Could you check a few things on this drawing? It's one solid part, dimensions in mm from its lowest x, y, z. A direction names the side the tool comes from. Round coordinates to 2 decimals unless told otherwise and drop trailing zeros. Write each loop counter-clockwise with the first axis right and the second up, starting at its lowest first coordinate (ties: lowest second). Pieces come first, ordered by that corner, then holes. Notation, with made-up numbers: M 44,-11 L 97,-11 A5 ccw 97,-4 Z; hole C 62.5,74 d4. An arc over 180 degrees is marked long. One line per item, written item: value. Start each with the question number.
(1) I want a section at B-B on z = 46. Please give me the cut outline in (x, y), and give its area (3 significant figures).
(2) I'm going to push flat-ended pins straight in: pin 1 Ø12.5 at (y, z) = (17, 46) entering from +X; pin 2 Ø2 at (x, y) = (60, 46.5) entering from +Z. Where does each tip first touch, or does it pass through?
(3) Which directions (+Z, -Z, +X, -X, +Y, -Y) give clear straight access to the entire face, cutting with the end or side of a thin tool? Please do the marked faces 1, 2 and 3.
(4) I want a section at D-D on z = 131. Please give me the cut outline in (x, y) (1 decimal).
(5) Thinking about a two-plate mould opening in Z: for the marked faces 4, 5 and 6, which applies, released by +Z, released by -Z, zero draft, split by the parting line, or undercut?
(6) I want a section at A-A on y = 95. Please give me the cut outline in (x, z).
(7) If I drill on L1, parallel to X at y = 68, z = 16; L2, parallel to Z at x = 15, y = 44.5 (1 decimal); L3, parallel to Z at x = 20, y = 40.5 (1 decimal), over which ranges is the centre line in solid material (lowest first)?
(8) I want a section at C-C on x = 84. Please give me the cut outline in (y, z), and give its area (3 significant figures).
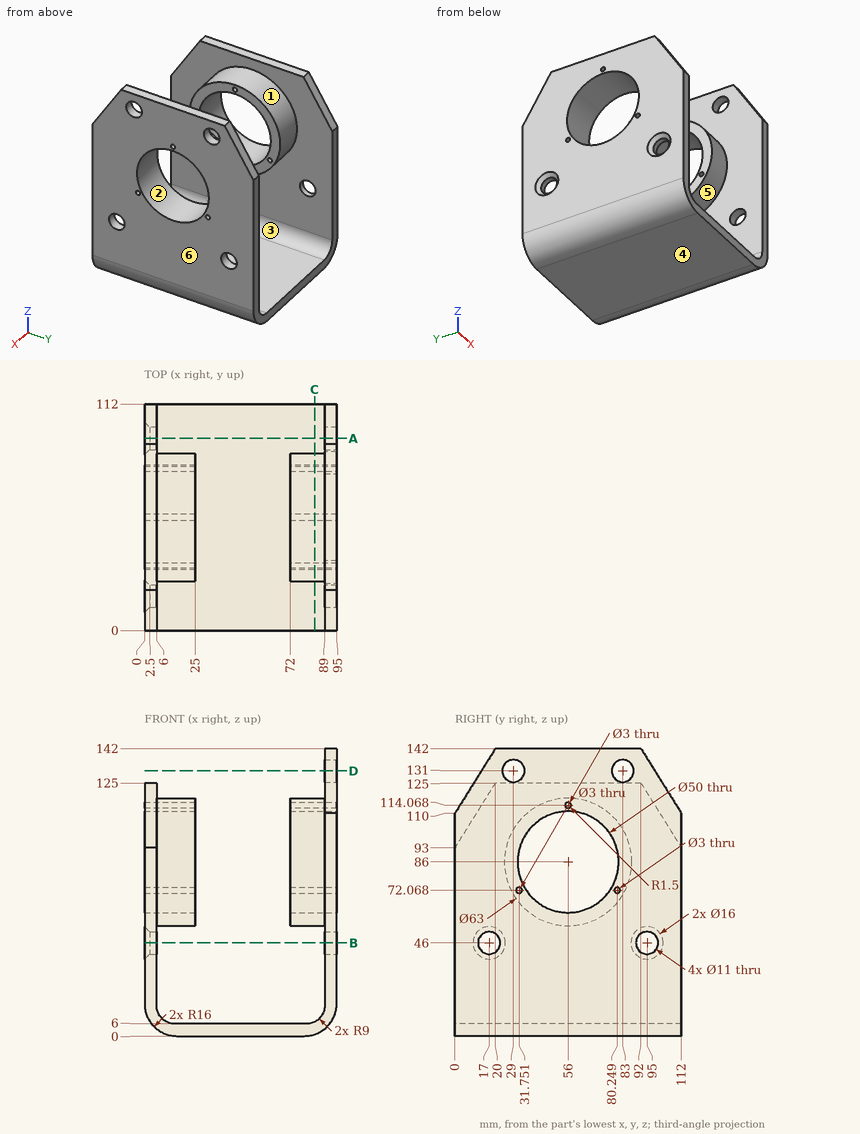
Found:
1. outline: M 0,0 L 6,0 L 6,11.5 L 2.5,11.5 L 0,9 Z; M 0,25 L 2.5,22.5 L 6,22.5 L 6,89.5 L 2.5,89.5 L 0,87 Z; M 0,103 L 2.5,100.5 L 6,100.5 L 6,112 L 0,112 Z; M 89,0 L 95,0 L 95,11.5 L 89,11.5 Z; M 89,22.5 L 95,22.5 L 95,89.5 L 89,89.5 Z; M 89,100.5 L 95,100.5 L 95,112 L 89,112 Z
1. area: 1,070 mm²
2. pin 1: stops at x = 95
2. pin 2: stops at z = 6
3. face 1: none
3. face 2: +X, -X
3. face 3: +Y, -Y
4. outline: M 89,13.1 L 95,13.1 L 95,23.5 L 89,23.5 Z; M 89,34.5 L 95,34.5 L 95,77.5 L 89,77.5 Z; M 89,88.5 L 95,88.5 L 95,98.9 L 89,98.9 Z
5. face 4: released by -Z
5. face 5: undercut
5. face 6: zero draft
6. outline: M 0,16 A16 ccw 16,0 L 79,0 A16 ccw 95,16 L 95,40.5 L 89,40.5 L 89,15 A9 cw 80,6 L 15,6 A9 cw 6,15 L 6,40.5 L 2.5,40.5 L 0,38 Z; M 0,54 L 2.5,51.5 L 6,51.5 L 6,120.2 L 0,120.2 Z; M 89,51.5 L 95,51.5 L 95,137.2 L 89,137.2 Z
7. L1: x = 0 to 6, 89 to 95
7. L2: z = 0 to 6, 56.7 to 63.8, 108.2 to 115.3
7. L3: z = 0 to 6, 58.6 to 66.4, 105.6 to 113.4
8. outline: M 0,0.8 L 112,0.8 L 112,6.94 L 0,6.94 Z; C 56,86 d63; hole C 31.75,72.07 d3; hole C 56,86 d50; hole C 56,114.07 d3; hole C 80.25,72.07 d3
8. area: 1,820 mm²
